The model under review builds one solid part; all positions refer to its coordinate system, in mm. Coordinates: 2 decimals unless noted, no trailing zeros. Write each loop counter-clockwise with the first axis right and the second up, starting at its lowest first coordinate (ties: lowest second). Pieces come first, ordered by that corner, then holes.
```python
from build123d import *

# Parameters (mm, degrees)
F0_W     = 127
F0_H     = 127
F1_DEPTH = 76.2
F3_DEPTH = 330.2
F4_W     = 127
F4_H     = 76.2
F4_R     = 12.7
F5_DEPTH = 127


with BuildPart() as f1:
    # F0 (on Top) → F1 (new body)
    with BuildSketch(Plane.XY):
        with Locations((-16.172883, 4.04909)):
            Rectangle(F0_W, F0_H)
    extrude(amount=F1_DEPTH)

    # F2 (on face) → F3 (join)
    with BuildSketch(Plane.YZ.offset(47.327117)):
        with BuildLine():
            ThreePointArc((-8.65091, 38.1), (4.04909, 25.4), (16.74909, 38.1))
            ThreePointArc((16.74909, 38.1), (4.04909, 50.8), (-8.65091, 38.1))
        make_face()
    extrude(amount=F3_DEPTH)

    # F4 (on face) → F5 (join)
    with BuildSketch(Plane.YZ.offset(377.527117)):
        with Locations((4.04909, 38.1)):
            Rectangle(F4_W, F4_H)
        with Locations((4.04909, 38.1)):
            Circle(F4_R, mode=Mode.SUBTRACT)
        with Locations((4.04909, 38.1)):
            Circle(F4_R)
    extrude(amount=F5_DEPTH)


solid = f1.part
```
Item 1: For pin 1 (8 mm diameter, centred on x = 276, y = 16, fed in from +Z); pin 2 (10 mm diameter, centred on x = 199, z = 40.5, fed in from -Y), all flat-tipped, find the tip position at first contact; note any pin that passes through.
Solved:
pin 1: stops at z = 48
pin 2: stops at y = -8.65
Item 2: Mouldability with a two-part tool opening along X and no side actions: class faces 1 (the face through (504.527, 3, 39)), 2 (the face through (210.116, 10.877, 48.809)), 3 (the face through (440, 3, 76.2)) as pulls with the +X half, pulls with the -X half, needs draft (parallel to the pull), parting line crosses it, or undercut.
Solved:
face 1: pulls with the +X half
face 2: undercut
face 3: needs draft
Item 3: To check wall thickness, follow line 1 along X through (y, z) = (6, 55.5); line 2 along Y through (x, z) = (200, 37); line 3 along Y through (x, z) = (137, 49.5). State the ranges of each line that lie inside material, in increasing order.
Solved:
line 1: x = -79.67 to 47.33, 377.53 to 504.53
line 2: y = -8.6 to 16.7
line 3: y = -1.55 to 9.65
Item 4: Take a section at B-B, the plane y = -36.5. Write out the cut boundary in (x, z), plus the area to 3 significant figures.
Solved:
outline: (-79.67, 0) - (47.33, 0) - (47.33, 76.2) - (-79.67, 76.2) - close; (377.53, 0) - (504.53, 0) - (504.53, 76.2) - (377.53, 76.2) - close
area: 19,400 mm2
Item 5: Take a section at D-D, the plane y = 10. Write out the cut boundary in (x, z).
Solved:
outline: (-79.67, 0) - (47.33, 0) - (47.33, 26.88) - (377.53, 26.88) - (377.53, 0) - (504.53, 0) - (504.53, 76.2) - (377.53, 76.2) - (377.53, 49.32) - (47.33, 49.32) - (47.33, 76.2) - (-79.67, 76.2) - close
Item 6: Take a section at A-A, the plane z = 8.5. Write out the cut boundary in (x, y), plus the area to 3 significant figures.
Solved:
outline: (-79.67, -59.45) - (47.33, -59.45) - (47.33, 67.55) - (-79.67, 67.55) - close; (377.53, -59.45) - (504.53, -59.45) - (504.53, 67.55) - (377.53, 67.55) - close
area: 32,300 mm2
Item 7: Take a section at C-C, the plane z = 38.1. Write out the cut boundary in (x, y).
Solved:
outline: (-79.67, -59.45) - (47.33, -59.45) - (47.33, -8.65) - (377.53, -8.65) - (377.53, -59.45) - (504.53, -59.45) - (504.53, 67.55) - (377.53, 67.55) - (377.53, 16.75) - (47.33, 16.75) - (47.33, 67.55) - (-79.67, 67.55) - close
